Work out the finished part from the listing and answer in its coordinate system (mm). Face numbers are marked on the shaded views. A direction names the side the tool comes from. Round coordinates to 2 decimals unless told otherwise and drop trailing zeros. Order: outer loops, then holes, each group sorted by start corner. A loop starts at its lowest first (then second) coordinate and runs counter-clockwise, first axis right, second up. Notation, with made-up numbers: (73, 39.5) - (121, 39.5) arc R20 ccw to (121, 65.5) - close; hole circle Ø1 at (64, 12). An arc over 180 degrees is marked (long way). Use one line per item in the form item = value. Start each with the question number.
Q1. The part is cut by section C-C on y = -88.5. Determine the outline of the cut face in (x, z), plus the area to 3 significant figures.
Q2. The part is cut by section B-B on y = -69. Determine the outline of the cut face in (x, z).
Q3. Find the intervals of material crossed by line 1 (Z direction, x = 13, y = -94.5); line 2 (Z direction, x = -23.5, y = -65); line 3 (Z direction, x = 45, y = -14), in increasing order. Write a range as [from, to].
Q4. The part is cut by section D-D on z = -31. Determine the outline of the cut face in (x, y), plus the area to 3 significant figures.
Q5. Which of the six approach directions +Z, -Z, +X, -X, +Y, -Y give full straight-line access (tool end or side, diameter ignored) to the marked faces 4, 5, 6, 7 and 8?
Q6. The part is cut by section A-A on z = -20. State how many separate pieces and enclosed holes the cut face has, plus the area to 3 significant figures.
Q7. Given P1, Ø5.5, axis at x = -35, y = 19.5, coming from the -Z side; P2, Ø4, axis at x = -35.5, y = -90, coming from the -Z side; P3, Ø2, axis at y = -6.5, z = -6.5, coming from the +X side; P4, Ø12, axis at x = -50, z = -39, coming from the -Y side (1 decimal), each flat-ended and moving along its own axis, determine where each tip first touches the part or whether it passes through.
Q8. For a pull along X with two mould halves and no side action, classify the marked faces 1, 2 and 3 as +X half, -X half, draft (parallel to the pull), parting line (faces both ways), or undercut.
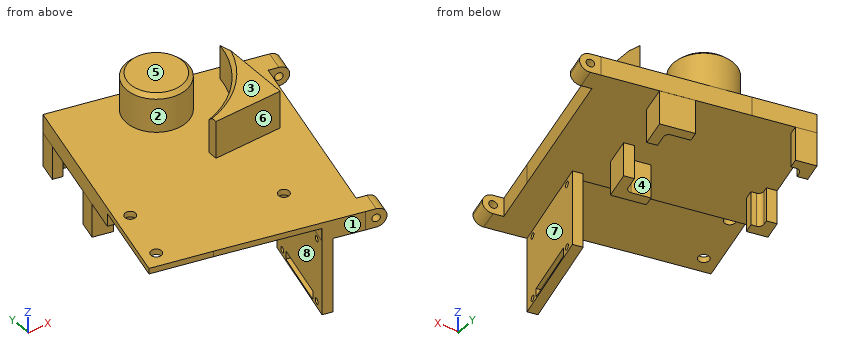
from build123d import *

# Parameters (mm, degrees)
SKETCH_1_R               = 15.75
EXTRUDE_1_DEPTH          = 20
EXTRUDE_1_2_DEPTH        = 20
EXTRUDE_5_DEPTH          = 10
CHAMFER_3_SIZE           = 2
SKETCH_18_W              = 10
SKETCH_18_H              = 10
EXTRUDE_6_DEPTH          = 10
CUT_EXTRUDE_1_DEPTH      = 148.860951012
CUT_EXTRUDE_1_DEPTH_BACK = 148.860951012
SKETCH_19_R              = 2
FILLET_2_R               = 5
EXTRUDE_7_DEPTH          = 10
CUT_EXTRUDE_2_DEPTH      = 7
SKETCH_23_R              = 2.75
CUT_EXTRUDE_3_DEPTH      = 7
EXTRUDE_9_DEPTH          = 18
FILLET_3_R               = 2.5
SKETCH_28_W              = 5
SKETCH_28_H              = 40
EXTRUDE_10_DEPTH         = 50
SKETCH_29_R              = 1.5
SKETCH_29_W              = 30
SKETCH_29_H              = 4.494622667
CUT_EXTRUDE_4_DEPTH      = 50


with BuildPart() as part:
    # Sketch 1 → Extrude 1 (new body)
    with BuildSketch(Plane(origin=(0, 0, 0), x_dir=(0, 1, 0), z_dir=(0, 0, 1))):
        with Locations(Location((0, 0, 0), (0, 0, 270))):
            Circle(SKETCH_1_R)
    extrude(amount=EXTRUDE_1_DEPTH)



with BuildPart() as body_2:
    # Sketch 1 → Extrude 1 2 (new body)
    with BuildSketch(Plane(origin=(0, 0, 0), x_dir=(0, 1, 0), z_dir=(0, 0, 1))):
        with BuildLine():
            ThreePointArc((0.501055918, -34.316325355), (-23.297606239, -22.583389768), (-37.227021319, 0))
            Line((-37.227021319, 0), (-42, 0))
            Line((-42, 0), (-42, -34.316325355))
            Line((-42, -34.316325355), (0.501055918, -34.316325355))
        make_face()
    extrude(amount=EXTRUDE_1_2_DEPTH)


with BuildPart() as part_1:
    add(part.part)

    add(body_2.part)  # Extrude 5 merges body 2
    # Sketch 17 → Extrude 5 (add)
    with BuildSketch(Plane(origin=(0, 0, 0), x_dir=(-1, 0, 0), z_dir=(0, 0, -1))):
        Polygon((-56.448813006, 2.157894853), (-37.030930328, -75.722978764), (-28.611757259, -109.490437583), (39.152120893, -91.926923446), (30.889770512, -58.788446072), (11.471887833, 19.092427545), align=None)
    extrude(amount=EXTRUDE_5_DEPTH)

    # Chamfer 3
    chamfer_3_edges = [part_1.edges().sort_by_distance(p)[0] for p in [
        (22.583389768, -23.297606239, 20),
        (-15.75, 0, 20),
    ]]
    chamfer(chamfer_3_edges, length=CHAMFER_3_SIZE)

    # Sketch 18 → Extrude 6 (add)
    with BuildSketch(Plane(origin=(52.63854315, -13.124262836, 0), x_dir=(0.24192189559966906, 0.9702957262759961, 0), z_dir=(0.9702957262759961, -0.24192189559966906, 0))):
        with Locations((-94.316293102, -5)):
            Rectangle(SKETCH_18_W, SKETCH_18_H)
        with Locations((10.75, -5)):
            Rectangle(SKETCH_18_W, SKETCH_18_H)
    extrude(amount=EXTRUDE_6_DEPTH)

    # Sketch 19 → Cut-Extrude 1 (cut, two sides: drawn at the far end of the back side and taken through both)
    with BuildSketch(Plane(origin=(-24.026785891, -96.366174746, 0), x_dir=(0.9702957262759961, -0.24192189559966903, 0), z_dir=(-0.24192189559966903, -0.9702957262759961, 0)).offset(-CUT_EXTRUDE_1_DEPTH_BACK)):
        with Locations((59.25, -5)):
            Circle(SKETCH_19_R)
    extrude(amount=CUT_EXTRUDE_1_DEPTH + CUT_EXTRUDE_1_DEPTH_BACK, mode=Mode.SUBTRACT)

    # Fillet 2
    fillet_2_edges = [part_1.edges().sort_by_distance(p)[0] for p in [
        (64.942160791, -5.112802735, -10),
        (64.942160791, -5.112802735, 0),
        (39.524324, -107.058177907, -10),
        (39.524324, -107.058177907, 0),
    ]]
    fillet(fillet_2_edges, radius=FILLET_2_R - 0.0001)  # a hair under: the kernel refuses the full size

    # Sketch 21 → Extrude 7 (add)
    with BuildSketch(Plane(origin=(0, 0, -10), x_dir=(1, 0, 0), z_dir=(0, 0, -1))):
        Polygon((-11.471887833, -19.092427545), (-39.152120893, 91.926923446), (-68.260992681, 84.669266578), (-40.580759621, -26.350084413), align=None)
    extrude(amount=-EXTRUDE_7_DEPTH)

    # Sketch 22 → Cut-Extrude 2 (cut)
    with BuildSketch(Plane(origin=(0, 0, -10), x_dir=(1, 0, 0), z_dir=(0, 0, -1))):
        Polygon((-68.260992681, 84.669266578), (-57.374507379, 41.005958895), (20.249150723, 60.359710543), (9.362665421, 104.023018226), (4.374510381, 124.029415356), (-73.249147721, 104.675663708), align=None)
    extrude(amount=-CUT_EXTRUDE_2_DEPTH, mode=Mode.SUBTRACT)

    # Sketch 23 → Cut-Extrude 3 (cut)
    with BuildSketch(Plane(origin=(0, 0, -3), x_dir=(1, 0, 0), z_dir=(0, 0, -1))):
        with Locations(Location((8.49768178, 78.557319663, 0), (0, 0, 180))):
            Circle(SKETCH_23_R)
        with Locations(Location((-52.638773407, 50.946925838, 0), (0, 0, 180))):
            Circle(SKETCH_23_R)
        with Locations(Location((-59.412586484, 78.115206174, 0), (0, 0, 180))):
            Circle(SKETCH_23_R)
    extrude(amount=-CUT_EXTRUDE_3_DEPTH, mode=Mode.SUBTRACT)

    # Sketch 27 → Extrude 9 (add)
    with BuildSketch(Plane(origin=(0, 0, -10), x_dir=(1, 0, 0), z_dir=(0, 0, -1))):
        Polygon((-42.999978577, -16.64712715), (-38.148499946, -15.437517672), (-36.938890468, -20.288996303), (-32.087411837, -19.079386825), (-30.877802359, -23.930865457), (-40.580759621, -26.350084413), align=None)
        Polygon((-47.341531979, 21.433719927), (-42.490053347, 22.643329405), (-43.699662825, 27.494808036), (-53.402620088, 25.07558908), (-50.983401132, 15.372631817), (-46.131922501, 16.582241295), align=None)
        Polygon((1.221618851, 38.694941482), (17.42896793, 42.735887459), (20.908348254, 28.780855193), (16.056869623, 27.571245715), (13.787098777, 36.674799349), (2.431228329, 33.84346285), align=None)
        Polygon((26.870688445, 4.724510909), (22.019209813, 3.514901431), (24.148746591, -5.026204076), (12.792876144, -7.857540575), (14.002485622, -12.709019206), (30.175814481, -8.676555422), align=None)
    extrude(amount=EXTRUDE_9_DEPTH)

    # Fillet 3
    fillet_3_edges = [part_1.edges().sort_by_distance(p)[0] for p in [
        (-36.938890468, 20.288996303, -19),
        (13.787098777, -36.674799349, -19),
        (24.148746591, 5.026204076, -19),
        (-47.341531979, -21.433719927, -19),
    ]]
    fillet(fillet_3_edges, radius=FILLET_3_R)

    # Sketch 28 → Extrude 10 (add)
    with BuildSketch(Plane(origin=(-24.791009663, -95.649136326, 0), x_dir=(0.9680138959056901, -0.25089658693072686, 0), z_dir=(-0.25089658693072686, -0.9680138959056901, 0))):
        with Locations((37.666498149, -30)):
            Rectangle(SKETCH_28_W, SKETCH_28_H)
    extrude(amount=-EXTRUDE_10_DEPTH)

    # Sketch 29 → Cut-Extrude 4 (cut)
    with BuildSketch(Plane(origin=(38.881728358, -10.077637295, 0), x_dir=(0.25089658693072686, 0.9680138959056901, 0), z_dir=(0.9680138959056901, -0.25089658693072686, 0))):
        with Locations((-54.809672806, -47)):
            Circle(SKETCH_29_R)
        with Locations((-92.809672806, -47)):
            Circle(SKETCH_29_R)
        with Locations((-92.809672806, -13)):
            Circle(SKETCH_29_R)
        with Locations((-54.809672806, -13)):
            Circle(SKETCH_29_R)
        with Locations((-73.809672806, -46.863560509)):
            Rectangle(SKETCH_29_W, SKETCH_29_H)
    extrude(amount=-CUT_EXTRUDE_4_DEPTH, mode=Mode.SUBTRACT)


solid = part_1.part
Found:
q1.outline = (-52.9, -3) - (13.23, -3) - (13.23, -10) - (13.39, -10) - (13.39, -44.62) - (18.56, -44.62) - (18.56, -10) - (33.85, -10) - (33.85, 0) - (-52.9, 0) - close; (13.39, -50) - (18.56, -50) - (18.56, -49.11) - (13.39, -49.11) - close
q1.area = 588 mm²
q2.outline = (-64.35, -3) - (18.09, -3) - (18.09, -10) - (18.44, -10) - (18.44, -44.62) - (23.61, -44.62) - (23.61, -10) - (38.71, -10) - (38.71, 0) - (-64.35, 0) - close; (18.44, -50) - (23.61, -50) - (23.61, -49.11) - (18.44, -49.11) - close
q3.line_1 = [-50, -49.11], [-44.62, 0]
q3.line_2 = [-3, 0]
q3.line_3 = [-10, 0]
q4.outline = (9.25, -104.47) - (14.09, -105.73) - (26.64, -57.33) - (21.8, -56.07) - close
q4.area = 250 mm²
q5.face_4 = -Z, +Y
q5.face_5 = +Z, +X, -X, +Y, -Y
q5.face_6 = +Z, +X, -X, -Y
q5.face_7 = -Z, +X, -Y
q5.face_8 = -Z, -X
q6.separate_pieces = 5
q6.enclosed_holes = 0
q6.area = 663 mm²
q7.P1 = -28
q7.P2 = -3
q7.P3 = 64.71
q7.P4 = through
q8.face_1 = -X half
q8.face_2 = undercut
q8.face_3 = draft
